from build123d import *

# Parameters (mm, degrees)
BOSS_EXTRUDE1_DEPTH = 19.05
FILLET1_R           = 76.2
FILLET2_R           = 19.05


with BuildPart() as part:
    # Sketch1 → Boss-Extrude1 (new body)
    with BuildSketch(Plane.XY):
        Polygon((-222.25, -177.8), (222.25, -177.8), (222.25, -29.36875), (180.975, -29.36875), (180.975, 29.36875), (222.25, 29.36875), (222.25, 177.8), (-222.25, 177.8), align=None)
        with BuildLine():
            Line((-194.4624, 15.08125), (-180.1749, 15.08125))
            ThreePointArc((-180.1749, 15.08125), (-165.09365, 0), (-180.1749, -15.08125))
            Line((-180.1749, -15.08125), (-194.4624, -15.08125))
            ThreePointArc((-194.4624, -15.08125), (-209.54365, 0), (-194.4624, 15.08125))
        make_face(mode=Mode.SUBTRACT)
        with BuildLine():
            Line((209.55, -134.9248), (209.55, -149.225))
            ThreePointArc((209.55, -149.225), (195.2625, -163.5125), (180.975, -149.225))
            Line((180.975, -149.225), (180.975, -134.9248))
            ThreePointArc((180.975, -134.9248), (195.2625, -120.6373), (209.55, -134.9248))
        make_face(mode=Mode.SUBTRACT)
        with BuildLine():
            Line((209.55, 134.9248), (209.55, 149.225))
            ThreePointArc((209.55, 149.225), (195.2625, 163.5125), (180.975, 149.225))
            Line((180.975, 149.225), (180.975, 134.9248))
            ThreePointArc((180.975, 134.9248), (195.2625, 120.6373), (209.55, 134.9248))
        make_face(mode=Mode.SUBTRACT)
    extrude(amount=BOSS_EXTRUDE1_DEPTH)

    # Fillet1
    fillet1_edges = [part.edges().sort_by_distance(p)[0] for p in [
        (-222.25, -177.8, 9.525),
        (-222.25, 177.8, 9.525),
    ]]
    fillet(fillet1_edges, radius=FILLET1_R)

    # Fillet2
    fillet2_edges = [part.edges().sort_by_distance(p)[0] for p in [
        (222.25, -177.8, 9.525),
        (222.25, 177.8, 9.525),
    ]]
    fillet(fillet2_edges, radius=FILLET2_R)


solid = part.part
Verification items for the finished model (mm, model axes). A direction names the side the tool comes from. Round coordinates to 2 decimals unless told otherwise and drop trailing zeros. Loops run counter-clockwise (first coordinate to the right, second up) from the corner with the lowest first, then second, coordinate; pieces in that order, holes last. Notation, with made-up numbers: (71.5, 19) - (91.5, 19) arc R31 ccw to (91.5, 58) - close; hole circle Ø9 at (48, -38). An arc over 180 degrees is marked (long way). Use a Markdown table: item, result. Add a question column.
1. Section check A-A, the plane y = 0. Record the boundary of the cut face in (x, z) (3 decimals), plus the area to 3 significant figures.
2. Gauge pin test, flat ends, axial feed: pin 1 (7 mm diameter, centred on y = -144.5, z = 13, fed in from -X); pin 2 (1.5 mm diameter, centred on y = -9.5, z = 13, fed in from +X) (3 decimals); pin 3 (5 mm diameter, centred on y = 106, z = 10.5, fed in from -X). Record the tip position at first contact, or that the pin passes through.
3. Access from +Z, -Z, +X, -X, +Y, -Y to the whole of each face (thin tool, end or side, straight path). Record for faces 1 (the face through (201, 29.369, 9)), 2 (the face through (31, 177.8, 9)), 3 (the face through (194.95, -120.64, 9.39)).
4. Release check for a two-part mould opening along Y. For faces 4 (the face through (-200.521, 154.886, 9.658)), 5 (the face through (-187, -15.081, 9)), 6 (the face through (-3, 2, 0)) record: released by +Y, released by -Y, zero draft, split by the parting line, or undercut.
5. Section check B-B, the plane z = 12.25. Give the number of separate pieces and of enclosed holes in the cut face, plus the area to 3 significant figures.
6. Thickness scan on probe 1 along Y at (x, z) = (185, 3.75); probe 2 along Y at (x, z) = (199.5, 8.75); probe 3 along X at (y, z) = (-0.5, 1) (3 decimals). Record the ranges inside material, lowest first. Write a range as [from, to].
Checks:
| question | item | result |
|---|---|---|
| 1 | outline | (-222.25, 0) - (-209.544, 0) - (-209.544, 19.05) - (-222.25, 19.05) - close; (-165.094, 0) - (180.975, 0) - (180.975, 19.05) - (-165.094, 19.05) - close |
| 1 | area | 6,830 mm^2 |
| 2 | pin 1 | stops at x = -211.27 |
| 2 | pin 2 | stops at x = 180.975 |
| 2 | pin 3 | stops at x = -222.23 |
| 3 | face 1 | +Z, -Z, +X |
| 3 | face 2 | +Z, -Z, +X, -X, +Y |
| 3 | face 3 | +Z, -Z |
| 4 | face 4 | released by +Y |
| 4 | face 5 | undercut |
| 4 | face 6 | zero draft |
| 5 | separate pieces | 1 |
| 5 | enclosed holes | 3 |
| 5 | area | 150,000 mm^2 |
| 6 | probe 1 | y = [-177.8, -159.17], [-124.98, -29.37], [29.37, 124.98], [159.17, 177.8] |
| 6 | probe 2 | y = [-177.8, -162.87], [-121.28, -29.37], [29.37, 121.28], [162.87, 177.8] |
| 6 | probe 3 | x = [-222.25, -209.535], [-165.102, 180.975] |
